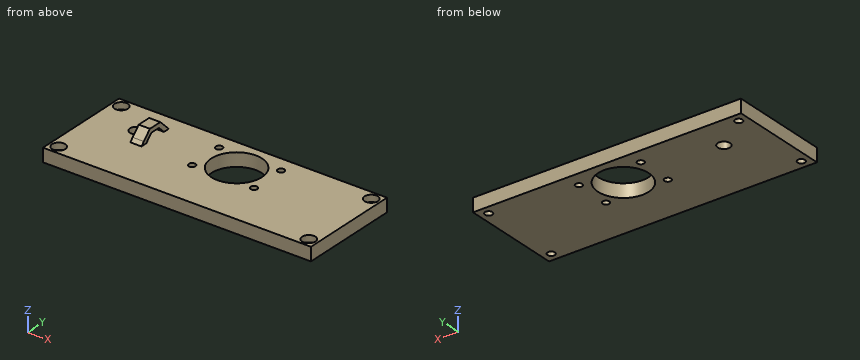
```python
from build123d import *

# Parameters (mm, degrees)
SKETCH1_W           = 120
SKETCH1_H           = 45
SKETCH1_R           = 11.3625
SKETCH1_R_2         = 1.65
SKETCH1_R_3         = 1.5
BOSS_EXTRUDE1_DEPTH = 6
CUT_EXTRUDE1_START  = -3
SKETCH2_R           = 3
SKETCH2_R_2         = 1.65
CUT_EXTRUDE1_DEPTH  = 3
SKETCH3_R           = 2.75
CUT_EXTRUDE2_DEPTH  = 129.300428682
BOSS_EXTRUDE2_START = -22.5
BOSS_EXTRUDE2_DEPTH = 5


with BuildPart() as part:
    # Sketch1 → Boss-Extrude1 (new body)
    with BuildSketch(Plane.XY):
        with Locations((60, 22.5)):
            Rectangle(SKETCH1_W, SKETCH1_H)
        with Locations((64, 30)):
            Circle(SKETCH1_R, mode=Mode.SUBTRACT)
        with Locations((4, 41)):
            Circle(SKETCH1_R_2, mode=Mode.SUBTRACT)
        with Locations(Location((4, 4, 0), (0, 0, 180))):
            Circle(SKETCH1_R_2, mode=Mode.SUBTRACT)
        with Locations(Location((116, 41, 0), (0, 0, 180))):
            Circle(SKETCH1_R_2, mode=Mode.SUBTRACT)
        with Locations((116, 4)):
            Circle(SKETCH1_R_2, mode=Mode.SUBTRACT)
        with Locations((50.143593539, 38)):
            Circle(SKETCH1_R_3, mode=Mode.SUBTRACT)
        with Locations(Location((50.143593539, 22, 0), (0, 0, 180))):
            Circle(SKETCH1_R_3, mode=Mode.SUBTRACT)
        with Locations((77.856406461, 22)):
            Circle(SKETCH1_R_3, mode=Mode.SUBTRACT)
        with Locations(Location((77.856406461, 38, 0), (0, 0, 180))):
            Circle(SKETCH1_R_3, mode=Mode.SUBTRACT)
    extrude(amount=BOSS_EXTRUDE1_DEPTH)

    # Sketch2 → Cut-Extrude1 (cut)
    # profile 1 of 4: a face of its own
    with BuildSketch(Plane.XY.offset(6).offset(CUT_EXTRUDE1_START)):
        with Locations((4, 41)):
            Circle(SKETCH2_R)
        with Locations((4, 41)):
            Circle(SKETCH2_R_2, mode=Mode.SUBTRACT)
    # profile 2 of 4: a face of its own
    with BuildSketch(Plane.XY.offset(6).offset(CUT_EXTRUDE1_START)):
        with Locations((4, 4)):
            Circle(SKETCH2_R)
        with Locations(Location((4, 4, 0), (0, 0, 180))):
            Circle(SKETCH2_R_2, mode=Mode.SUBTRACT)
    # profile 3 of 4: a face of its own
    with BuildSketch(Plane.XY.offset(6).offset(CUT_EXTRUDE1_START)):
        with Locations((116, 4)):
            Circle(SKETCH2_R)
        with Locations((116, 4)):
            Circle(SKETCH2_R_2, mode=Mode.SUBTRACT)
    # profile 4 of 4: a face of its own
    with BuildSketch(Plane.XY.offset(6).offset(CUT_EXTRUDE1_START)):
        with Locations((116, 41)):
            Circle(SKETCH2_R)
        with Locations(Location((116, 41, 0), (0, 0, 180))):
            Circle(SKETCH2_R_2, mode=Mode.SUBTRACT)
    extrude(amount=CUT_EXTRUDE1_DEPTH, mode=Mode.SUBTRACT)

    # Sketch3 → Cut-Extrude2 (cut, through all)
    with BuildSketch(Plane.XY.offset(6)):
        with Locations((19, 30)):
            Circle(SKETCH3_R)
    extrude(amount=-CUT_EXTRUDE2_DEPTH, mode=Mode.SUBTRACT)

    # Sketch4 → Boss-Extrude2 (add)
    with BuildSketch(Plane.ZY.offset(BOSS_EXTRUDE2_START)):
        Polygon((6, 35.25), (9, 32.25), (9, 27.75), (6, 24.75), (6, 21.921572875), (7.414213562, 23.335786438), (11, 26.921572875), (11, 33.078427125), (7.414213562, 36.664213562), (6, 38.078427125), align=None)
    extrude(amount=-BOSS_EXTRUDE2_DEPTH)


solid = part.part
```
Could you check a few things on this model? Use its own coordinates, in mm. Give positions to 0.01 mm unless a question says otherwise; leave off trailing zeros. Loops run counter-clockwise (first coordinate to the right, second up) from the corner with the lowest first, then second, coordinate; pieces in that order, holes last. Notation, with made-up numbers: (37, 55) - (66, 55) arc R14 ccw to (66, 76) - close; hole circle Ø6 at (60, 60). An arc over 180 degrees is marked (long way). Answer in a Markdown table with one row per item. Add a question column.
Q1. Please list where these lines run through material, in increasing order: L1, parallel to Y at x = 4, z = 4.95; L2, parallel to X at y = 5, z = 5.25; L3, parallel to Z at x = 26.5, y = 42.5. Write a range as from..to.
Q2. If we section it at C-C (z = 4.25): State how many separate pieces and enclosed holes the cut face has, plus the area to 3 significant figures.
Q3. If we section it at B-B (y = 4): List the corners of the cut face in (x, z) for me, plus the area to 3 significant figures.
Q4. If we section it at A-A (x = 19): List the corners of the cut face in (y, z) for me, plus the area to 3 significant figures.
Q5. For pin 1 (2 mm diameter, centred on x = 4, y = 4, fed in from -Z); pin 2 (3 mm diameter, centred on x = 5, y = 3.5, fed in from +Z); pin 3 (10 mm diameter, centred on x = 18, y = 38.5, fed in from +Z); pin 4 (2.5 mm diameter, centred on y = 29.5, z = 8.5, fed in from +X), each with a flat end and sliding along its axis, tell me the tip position at first contact or that it passes through.
Q6. If we section it at D-D (x = 116): List the corners of the cut face in (y, z) for me, plus the area to 3 significant figures.
The answers:
| question | item | result |
|---|---|---|
| 1 | L1 | y = 0..1, 7..38, 44..45 |
| 1 | L2 | x = 0..1.17, 6.83..113.17, 118.83..120 |
| 1 | L3 | z = 0..6 |
| 2 | separate pieces | 1 |
| 2 | enclosed holes | 10 |
| 2 | area | 4,830 mm^2 |
| 3 | outline | (0, 0) - (2.35, 0) - (2.35, 3) - (1, 3) - (1, 6) - (0, 6) - close; (5.65, 0) - (114.35, 0) - (114.35, 3) - (113, 3) - (113, 6) - (7, 6) - (7, 3) - (5.65, 3) - close; (117.65, 0) - (120, 0) - (120, 6) - (119, 6) - (119, 3) - (117.65, 3) - close |
| 3 | area | 664 mm^2 |
| 4 | outline | (0, 0) - (27.25, 0) - (27.25, 6) - (0, 6) - close; (32.75, 0) - (45, 0) - (45, 6) - (32.75, 6) - close |
| 4 | area | 237 mm^2 |
| 5 | pin 1 | passes through |
| 5 | pin 2 | stops at z = 3 |
| 5 | pin 3 | stops at z = 7.76 |
| 5 | pin 4 | stops at x = 27.5 |
| 6 | outline | (0, 0) - (2.35, 0) - (2.35, 3) - (1, 3) - (1, 6) - (0, 6) - close; (5.65, 0) - (39.35, 0) - (39.35, 3) - (38, 3) - (38, 6) - (7, 6) - (7, 3) - (5.65, 3) - close; (42.65, 0) - (45, 0) - (45, 6) - (44, 6) - (44, 3) - (42.65, 3) - close |
| 6 | area | 214 mm^2 |
